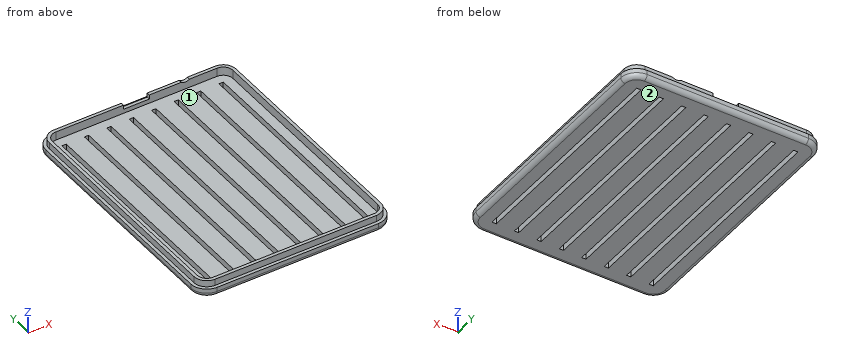
Autodesk Inventor part; units mm, degrees
ref_plane "YZ Plane" through (0, 0, 0) normal (1, 0, 0) x (0, 1, 0)
ref_plane "XZ Plane" through (0, 0, 0) normal (0, 1, 0) x (-1, 0, 0)
ref_plane "XY Plane" through (0, 0, 0) normal (0, 0, 1) x (1, 0, 0)
sketch "Sketch6" plane through (0, 0, 0) normal (0, 0, 1) x (1, 0, 0)
  arc A0 (83, 106.5858) -> (78.5858, 111) centre (78.5858, 106.5858) ccw
  line L0 (83, 106.5858) -> (83, 3.4142)
  arc A1 (78.5858, -1) -> (83, 3.4142) centre (78.5858, 3.4142) ccw
  line L1 (78.5858, -1) -> (3.4142, -1)
  arc A2 (-1, 3.4142) -> (3.4142, -1) centre (3.4142, 3.4142) ccw
  line L2 (-1, 3.4142) -> (-1, 106.5858)
  arc A3 (3.4142, 111) -> (-1, 106.5858) centre (3.4142, 106.5858) ccw
  line L3 (3.4142, 111) -> (78.5858, 111)
  arc A4 (86, 106.5858) -> (78.5858, 114) centre (78.5858, 106.5858) ccw
  line L4 (86, 106.5858) -> (86, 3.4142)
  arc A5 (78.5858, -4) -> (86, 3.4142) centre (78.5858, 3.4142) ccw
  line L5 (78.5858, -4) -> (3.4142, -4)
  arc A6 (-4, 3.4142) -> (3.4142, -4) centre (3.4142, 3.4142) ccw
  line L6 (-4, 3.4142) -> (-4, 106.5858)
  arc A7 (3.4142, 114) -> (-4, 106.5858) centre (3.4142, 106.5858) ccw
  line L7 (3.4142, 114) -> (78.5858, 114)
extrude "Extrusion4" add sketch "Sketch6" along normal blind 3 contours L0 A1 L1 A2 L2 A3 L3 A0 | L4 A5 L5 A6 L6 A7 L7 A4
sketch "Sketch7" plane through (0, 0, 3) normal (0, 0, 1) x (1, 0, 0)
  line L0 (83, 106.5858) -> (83, 3.4142)
  line L1 (-1, 3.4142) -> (-1, 106.5858)
  arc A0 (78.5858, -1) -> (83, 3.4142) centre (78.5858, 3.4142) ccw
  arc A1 (-1, 3.4142) -> (3.4142, -1) centre (3.4142, 3.4142) ccw
  line L2 (78.5858, -1) -> (3.4142, -1)
  line L3 (3.4142, 111) -> (78.5858, 111)
  arc A2 (3.4142, 111) -> (-1, 106.5858) centre (3.4142, 106.5858) ccw
  arc A3 (83, 106.5858) -> (78.5858, 111) centre (78.5858, 106.5858) ccw
  line L4 (-4, 106.5858) -> (-4, 3.4142)
  arc A4 (-4, 3.4142) -> (3.4142, -4) centre (3.4142, 3.4142) ccw
  line L5 (3.4142, -4) -> (78.5858, -4)
  arc A5 (78.5858, -4) -> (86, 3.4142) centre (78.5858, 3.4142) ccw
  line L6 (86, 3.4142) -> (86, 106.5858)
  arc A6 (86, 106.5858) -> (78.5858, 114) centre (78.5858, 106.5858) ccw
  line L7 (78.5858, 114) -> (3.4142, 114)
  arc A7 (3.4142, 114) -> (-4, 106.5858) centre (3.4142, 106.5858) ccw
  point P0 (0, 0)
  dimension "d17" = 3
extrude "Extrusion5" add sketch "Sketch7" along normal blind 4
sketch "Sketch8" plane through (0, 0, 7) normal (0, 0, 1) x (1, 0, 0)
  arc A0 (3.4142, 111) -> (-1, 106.5858) centre (3.4142, 106.5858) ccw
  line L0 (3.4142, 111) -> (78.5858, 111)
  arc A1 (83, 106.5858) -> (78.5858, 111) centre (78.5858, 106.5858) ccw
  line L1 (-1, 3.4142) -> (-1, 106.5858)
  line L2 (83, 106.5858) -> (83, 3.4142)
  arc A2 (-1, 3.4142) -> (3.4142, -1) centre (3.4142, 3.4142) ccw
  line L3 (78.5858, -1) -> (3.4142, -1)
  arc A3 (78.5858, -1) -> (83, 3.4142) centre (78.5858, 3.4142) ccw
  line L4 (-4, 106.5858) -> (-4, 3.4142)
  arc A4 (-4, 3.4142) -> (3.4142, -4) centre (3.4142, 3.4142) ccw
  line L5 (3.4142, -4) -> (78.5858, -4)
  arc A5 (78.5858, -4) -> (86, 3.4142) centre (78.5858, 3.4142) ccw
  line L6 (86, 3.4142) -> (86, 106.5858)
  arc A6 (86, 106.5858) -> (78.5858, 114) centre (78.5858, 106.5858) ccw
  line L7 (78.5858, 114) -> (3.4142, 114)
  arc A7 (3.4142, 114) -> (-4, 106.5858) centre (3.4142, 106.5858) ccw
  line L8 (-2.5, 106.5858) -> (-2.5, 3.4142)
  arc A8 (-2.5, 3.4142) -> (3.4142, -2.5) centre (3.4142, 3.4142) ccw
  line L9 (3.4142, -2.5) -> (78.5858, -2.5)
  arc A9 (78.5858, -2.5) -> (84.5, 3.4142) centre (78.5858, 3.4142) ccw
  line L10 (84.5, 3.4142) -> (84.5, 106.5858)
  arc A10 (84.5, 106.5858) -> (78.5858, 112.5) centre (78.5858, 106.5858) ccw
  line L11 (78.5858, 112.5) -> (3.4142, 112.5)
  arc A11 (3.4142, 112.5) -> (-2.5, 106.5858) centre (3.4142, 106.5858) ccw
  point P0 (0, 0)
  point P1 (0, 0)
  dimension "d20" = 3
  dimension "d21" = 1.5
extrude "Extrusion6" cut sketch "Sketch8" against normal blind 3 contours A7 L7 A6 L6 A5 L5 A4 L4
fillet "Fillet2" radius 2 8 edges at (-1.8284, 111.8284, 0) (-4, 55, 0) (-1.8284, -1.8284, 0) (41, -4, 0) (83.8284, -1.8284, 0) (86, 55, 0) (83.8284, 111.8284, 0) (41, 114, 0)
sketch "Sketch9" plane through (3.4142, 111, 3) normal (0, -1, 0) x (1, 0, 0)
  circle A0 centre (60.4216, 6.636) radius 3.25
  line L0 (31.5858, 6) -> (43.5858, 6)
  line L1 (43.5858, 6) -> (43.5858, 2)
  line L2 (43.5858, 2) -> (31.5858, 2)
  line L3 (31.5858, 2) -> (31.5858, 6)
  line L4 (31.5858, 6) -> (43.5858, 2) construction
  line L5 (43.5858, 6) -> (31.5858, 2) construction
  point P0 (37.5858, 4)
  dimension "d55" = 12
  dimension "d56" = 4
extrude "Extrusion7" cut sketch "Sketch9" against normal blind 3
sketch "Sketch11" plane through (0, 0, 3) normal (0, 0, 1) x (1, 0, 0)
  line L0 (3.4142, 3.4142) -> (5.4142, 3.4142)
  line L1 (5.4142, 3.4142) -> (5.4142, 106.5858)
  line L2 (5.4142, 106.5858) -> (3.4142, 106.5858)
  line L3 (3.4142, 106.5858) -> (3.4142, 3.4142)
  line L4 (13.8642, 3.4142) -> (15.8642, 3.4142)
  line L5 (15.8642, 3.4142) -> (15.8642, 106.5858)
  line L6 (15.8642, 106.5858) -> (13.8642, 106.5858)
  line L7 (13.8642, 106.5858) -> (13.8642, 3.4142)
  line L8 (24.3142, 3.4142) -> (26.3142, 3.4142)
  line L9 (26.3142, 3.4142) -> (26.3142, 106.5858)
  line L10 (26.3142, 106.5858) -> (24.3142, 106.5858)
  line L11 (24.3142, 106.5858) -> (24.3142, 3.4142)
  line L12 (34.7642, 3.4142) -> (36.7642, 3.4142)
  line L13 (36.7642, 3.4142) -> (36.7642, 106.5858)
  line L14 (36.7642, 106.5858) -> (34.7642, 106.5858)
  line L15 (34.7642, 106.5858) -> (34.7642, 3.4142)
  line L16 (45.2142, 3.4142) -> (47.2142, 3.4142)
  line L17 (47.2142, 3.4142) -> (47.2142, 106.5858)
  line L18 (47.2142, 106.5858) -> (45.2142, 106.5858)
  line L19 (45.2142, 106.5858) -> (45.2142, 3.4142)
  line L20 (55.6642, 3.4142) -> (57.6642, 3.4142)
  line L21 (57.6642, 3.4142) -> (57.6642, 106.5858)
  line L22 (57.6642, 106.5858) -> (55.6642, 106.5858)
  line L23 (55.6642, 106.5858) -> (55.6642, 3.4142)
  line L24 (66.1142, 3.4142) -> (68.1142, 3.4142)
  line L25 (68.1142, 3.4142) -> (68.1142, 106.5858)
  line L26 (68.1142, 106.5858) -> (66.1142, 106.5858)
  line L27 (66.1142, 106.5858) -> (66.1142, 3.4142)
  line L28 (76.5642, 3.4142) -> (78.5642, 3.4142)
  line L29 (78.5642, 3.4142) -> (78.5642, 106.5858)
  line L30 (78.5642, 106.5858) -> (76.5642, 106.5858)
  line L31 (76.5642, 106.5858) -> (76.5642, 3.4142)
  dimension "d57" = 2
  dimension "d60" = 10.45
extrude "Extrusion9" cut sketch "Sketch11" against normal blind 3
properties part number "CaseGroboyBack"
Model file for the job. Use its own axes, mm. Face numbers are marked on the shaded views. Coordinates: 2 decimals unless noted, no trailing zeros. Order: outer loops, then holes, each group sorted by start corner. A loop starts at its lowest first (then second) coordinate and runs counter-clockwise, first axis right, second up. Notation, with made-up numbers: (-8.5, 32) -> (14.5, 32) arc R15 cw to (14.5, 57) -> close; hole circle Ø3 at (-15, 18). An arc over 180 degrees is marked (long way). Return JSON: item names as keys, results as strings. Group by question number.
Item 1: Flat gauge pins, fed straight in: P1, Ø1.5, axis at y = 69, z = 1, coming from the -X side; P2, Ø1.5, axis at x = 42, z = 6, coming from the +Y side; P3, Ø1.6, axis at x = 40, y = 111.5, coming from the +Z side. Where does each tip first touch, or does it go through?
Item 2: Pull direction Y, two halves, no side cores. Call the marked faces 1 and 2: pulls with the +Y half, pulls with the -Y half, needs draft (parallel to the pull), parting line crosses it, or undercut.
Item 3: Saw through at B-B on y = 79. State how many separate pieces and enclosed holes the cut face has, then the cut area to 3 significant figures.
Item 4: Wall check: line 1 along X through (y, z) = (29, 3.75); line 2 along X through (y, z) = (13, 5.5); line 3 along Y through (x, z) = (56, 3.5). Give the ranges that are in metal, low to high. Write a range as [from, to].
Item 5: Saw through at A-A on x = 8.5. Write the cut outline in (y, z).
Values found:
{
 "1": {"P1": "stops at x = -3.98", "P2": "stops at y = -1", "P3": "stops at z = 5"},
 "2": {"face 1": "undercut", "face 2": "needs draft"},
 "3": {"separate pieces": "9", "enclosed holes": "0", "area": "235 mm2"},
 "4": {"line 1": "x = [-4, -1], [83, 86]", "line 2": "x = [-2.5, -1], [83, 84.5]", "line 3": "y = [-4, -1], [111, 114]"},
 "5": {"outline": "(-4, 2) arc R2 ccw to (-2, 0) -> (112, 0) arc R2 ccw to (114, 2) -> (114, 4) -> (112.5, 4) -> (112.5, 7) -> (111, 7) -> (111, 3) -> (-1, 3) -> (-1, 7) -> (-2.5, 7) -> (-2.5, 4) -> (-4, 4) -> close"}
}
